Read the model definition and answer for the solid it produces. Units are mm, in the model's axes. Give positions to 0.01 mm unless a question says otherwise; leave off trailing zeros. Write each loop counter-clockwise with the first axis right and the second up, starting at its lowest first coordinate (ties: lowest second). Pieces come first, ordered by that corner, then holes. Notation, with made-up numbers: (89, 67.25) -> (105, 67.25) arc R27 ccw to (105, 93.25) -> close; hole circle Ø11 at (23, 55). An arc over 180 degrees is marked (long way). Write item = value, one per line.
from build123d import *

# Parameters (mm, degrees)
ESTRUSIONE_ESTRUSIONE1_DEPTH = 6


with BuildPart() as part:
    # Schizzo1 → Estrusione-Estrusione1 (new body)
    with BuildSketch(Plane.XY):
        Polygon((6, -115.594034624), (0, -115.594034624), (0, -100.594034624), (6, -100.594034624), (6, -101.959034624), (13.28, -99.229034624), (13.28, -96.044034624), (6, -96.044034624), (0, -96.044034624), (0, -86.944034624), (6, -86.944034624), (13.28, -86.944034624), (13.28, -83.759034624), (6, -81.029034624), (6, -82.394034624), (0, -82.394034624), (0, -78.644034624), (-120, -78.644034624), (-120, -82.394034624), (-126, -82.394034624), (-126, -81.029034624), (-133.28, -83.759034624), (-133.28, -86.944034624), (-126, -86.944034624), (-120, -86.944034624), (-120, -96.044034624), (-126, -96.044034624), (-133.28, -96.044034624), (-133.28, -99.229034624), (-126, -101.959034624), (-126, -100.594034624), (-120, -100.594034624), (-120, -115.594034624), (-126, -115.594034624), (-126, -114.229034624), (-133.28, -116.959034624), (-133.28, -120.144034624), (-126, -120.144034624), (-120, -120.144034624), (-120, -129.244034624), (-126, -129.244034624), (-133.28, -129.244034624), (-133.28, -132.429034624), (-126, -135.159034624), (-126, -133.794034624), (-120, -133.794034624), (-120, -137.544034624), (0, -137.544034624), (0, -133.794034624), (6, -133.794034624), (6, -135.159034624), (13.28, -132.429034624), (13.28, -129.244034624), (6, -129.244034624), (0, -129.244034624), (0, -120.144034624), (6, -120.144034624), (13.28, -120.144034624), (13.28, -116.959034624), (6, -114.229034624), align=None)
        with BuildLine():
            Line((-72, -90.094034624), (-48, -90.094034624))
            ThreePointArc((-48, -90.094034624), (-30, -108.094034624), (-48, -126.094034624))
            Line((-48, -126.094034624), (-72, -126.094034624))
            ThreePointArc((-72, -126.094034624), (-90, -108.094034624), (-72, -90.094034624))
        make_face(mode=Mode.SUBTRACT)
    extrude(amount=ESTRUSIONE_ESTRUSIONE1_DEPTH)


solid = part.part
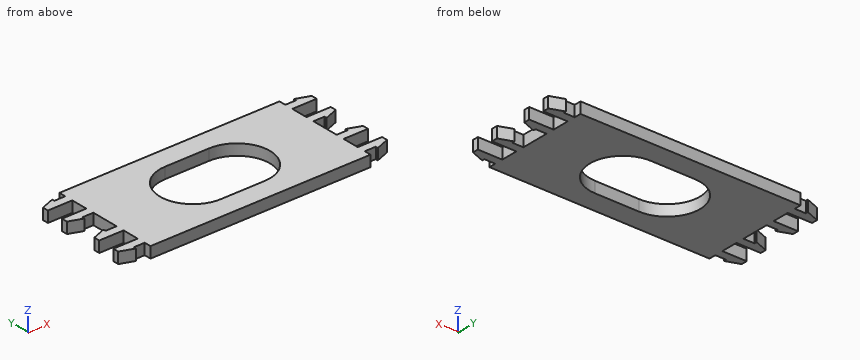
(1) Given P1, Ø1.8, axis at y = -109.5, z = 4, coming from the +X side; P2, Ø3, axis at x = -110, y = -86.5, coming from the -Z side; P3, Ø1.8, axis at x = -122.5, z = 2, coming from the +Y side; P4, Ø3, axis at x = -126, z = 3, coming from the +Y side, each flat-ended and moving along its own axis, determine where each tip first touches the part or whether it passes through.
Checks:
P1 = 0
P2 = 0
P3 = -82.39
P4 = -81.03
(2) Consider L1, parallel to Y at x = -125, z = 1.9; L2, parallel to X at y = -109, z = 3; L3, parallel to Y at x = 7, z = 3.45. Determine where each line is inside the solid, lowest interval first.
Checks:
L1 = -133.79 to -129.24, -120.14 to -115.59, -100.59 to -96.04, -86.94 to -82.39
L2 = -120 to -89.98, -30.02 to 0
L3 = -134.78 to -129.24, -120.14 to -114.6, -101.58 to -96.04, -86.94 to -81.4
(3) The part is cut by section A-A on x = -60.5. Determine the outline of the cut face in (y, z).
Checks:
outline = (-137.54, 0) -> (-126.09, 0) -> (-126.09, 6) -> (-137.54, 6) -> close; (-90.09, 0) -> (-78.64, 0) -> (-78.64, 6) -> (-90.09, 6) -> close
(4) The part is cut by section B-B on y = -111. Determine the outline of the cut face in (x, z).
Checks:
outline = (-120, 0) -> (-89.76, 0) -> (-89.76, 6) -> (-120, 6) -> close; (-30.24, 0) -> (0, 0) -> (0, 6) -> (-30.24, 6) -> close
